Part model, mm, in its own coordinate system. Face numbers are marked on the shaded views. A direction names the side the tool comes from. Give positions to 0.01 mm unless a question says otherwise; leave off trailing zeros. Order: outer loops, then holes, each group sorted by start corner. A loop starts at its lowest first (then second) coordinate and runs counter-clockwise, first axis right, second up. Notation, with made-up numbers: M -25.75,14 L 20.25,14 A17 ccw 20.25,32 Z; hole C 54.5,16 d9. An arc over 180 degrees is marked long. One line per question, with ' | ' between items.
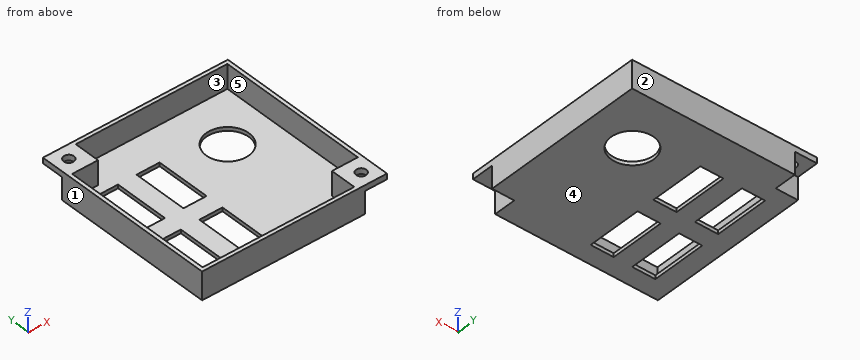
```python
from build123d import *

# Parameters (mm, degrees)
SKETCH_W        = 100
SKETCH_H        = 100
PAD_DEPTH       = 15
POCKET_DEPTH    = 13
SKETCH002_W     = 12
SKETCH002_H     = 12
POCKET001_DEPTH = 12
SKETCH003_R     = 2.75
POCKET002_DEPTH = 3
SKETCH004_R     = 11.5
SKETCH004_W     = 12.5
SKETCH004_H     = 29.5
POCKET003_DEPTH = 3


with BuildPart() as part:
    # Sketch → Pad (new body)
    with BuildSketch(Plane.XY):
        with Locations((50, 50)):
            Rectangle(SKETCH_W, SKETCH_H)
    extrude(amount=PAD_DEPTH)

    # Sketch001 → Pocket (cut)
    with BuildSketch(Plane.XY.offset(15)):
        Polygon((2, 2), (2, 84), (16, 84), (16, 98), (98, 98), (98, 16), (84, 16), (84, 2), align=None)
    extrude(amount=-POCKET_DEPTH, mode=Mode.SUBTRACT)

    # Sketch002 → Pocket001 (cut)
    with BuildSketch(Plane(origin=(0, 0, 0), x_dir=(1, 0, 0), z_dir=(0, 0, -1))):
        with Locations((94, -6)):
            Rectangle(SKETCH002_W, SKETCH002_H)
        with Locations((6, -94)):
            Rectangle(SKETCH002_W, SKETCH002_H)
    extrude(amount=-POCKET001_DEPTH, mode=Mode.SUBTRACT)

    # Sketch003 → Pocket002 (cut)
    with BuildSketch(Plane.XY.offset(15)):
        with Locations((7.5, 92.5)):
            Circle(SKETCH003_R)
        with Locations((92.5, 7.5)):
            Circle(SKETCH003_R)
    extrude(amount=-POCKET002_DEPTH, mode=Mode.SUBTRACT)

    # Sketch004 → Pocket003 (cut)
    with BuildSketch(Plane(origin=(0, 0, 0), x_dir=(1, 0, 0), z_dir=(0, 0, -1))):
        with Locations((74, -70)):
            Circle(SKETCH004_R)
        with Locations((16.25, -24.75)):
            Rectangle(SKETCH004_W, SKETCH004_H)
        with Locations((16.25, -64.25)):
            Rectangle(SKETCH004_W, SKETCH004_H)
        with Locations((38.75, -24.75)):
            Rectangle(SKETCH004_W, SKETCH004_H)
        with Locations((38.75, -64.25)):
            Rectangle(SKETCH004_W, SKETCH004_H)
    extrude(amount=-POCKET003_DEPTH, mode=Mode.SUBTRACT)


solid = part.part
```
1. Probe L1, parallel to Y at x = 7.5, z = 13.3; L2, parallel to Y at x = 92.5, z = 14.1; L3, parallel to X at y = 54.5, z = 5.5. List the from-to ranges inside material, lowest first. Write a range as from..to.
Worked out:
L1: y = 0..2, 84..89.75, 95.25..100 | L2: y = 0..4.75, 10.25..16, 98..100 | L3: x = 0..2, 98..100
2. Slice it at D-D on y = 70. Give the cut face in (x, z), then the cut area to 3 significant figures.
Worked out:
outline: M 0,0 L 10,0 L 10,2 L 2,2 L 2,15 L 0,15 Z; M 22.5,0 L 32.5,0 L 32.5,2 L 22.5,2 Z; M 45,0 L 62.5,0 L 62.5,2 L 45,2 Z; M 85.5,0 L 100,0 L 100,15 L 98,15 L 98,2 L 85.5,2 Z | area: 156 mm2
3. Tool access for the marked faces 4 and 5: list every direction of +Z, -Z, +X, -X, +Y, -Y with a clear straight run to the whole face (end or side of a thin tool).
Worked out:
face 4: -Z, +X, -X, +Y, -Y | face 5: +Z
4. Slice it at A-A on y = 7.5. Give the cut face in (x, z).
Worked out:
outline: M 0,0 L 88,0 L 88,12 L 89.75,12 L 89.75,15 L 84,15 L 84,2 L 2,2 L 2,15 L 0,15 Z; M 95.25,12 L 100,12 L 100,15 L 95.25,15 Z
5. Drop flat-ended pins along their axis: pin 1 (3.5 mm diameter, centred on y = 96, z = 9, fed in from -X); pin 2 (10 mm diameter, centred on x = 49, y = 43, fed in from +Z). Give the stop position or say it passes through.
Worked out:
pin 1: stops at x = 12 | pin 2: stops at z = 2
6. Mould opens along X. For the marked faces 1, 2 and 3 say: released by +X, released by -X, zero draft, split by the parting line, or undercut.
Worked out:
face 1: released by -X | face 2: zero draft | face 3: undercut
7. Slice it at C-C on z = 5.5. Give the cut face in (x, y), then the cut area to 3 significant figures.
Worked out:
outline: M 0,0 L 88,0 L 88,12 L 100,12 L 100,100 L 12,100 L 12,88 L 0,88 Z; hole M 2,2 L 84,2 L 84,16 L 98,16 L 98,98 L 16,98 L 16,84 L 2,84 Z | area: 888 mm2
8. Slice it at B-B on x = 74. Give the cut face in (y, z), then the cut area to 3 significant figures.
Worked out:
outline: M 0,0 L 58.5,0 L 58.5,2 L 2,2 L 2,15 L 0,15 Z; M 81.5,0 L 100,0 L 100,15 L 98,15 L 98,2 L 81.5,2 Z | area: 206 mm2
